```python
from build123d import *

# Parameters (mm, degrees)
FILETE1_R     = 2
CHANFRO1_SIZE = 0.5


with BuildPart() as part:
    # Esboço1 → Revolução1 (revolve)
    with BuildSketch(Plane.XY, mode=Mode.PRIVATE) as revolu_o1_sk:
        Polygon((0, 58.936157254), (12.5, 58.936157254), (12.5, 54.936157254), (6, 54.936157254), (6, 42.536157254), (4, 42.536157254), (4, 22.536157254), (1.75, 22.536157254), (1.75, 30.536157254), (0, 31.786157254), align=None)
    revolve(revolu_o1_sk.sketch.rotate(Axis((0, -51.524307863, 0), (0, 1, 0)), 90), axis=Axis((0, -51.524307863, 0), (0, 1, 0)))

    # Filete1
    filete1_edges = [part.edges().sort_by_distance(p)[0] for p in [
        (0, 54.936157254, 12.5),
        (0, 58.936157254, 12.5),
    ]]
    fillet(filete1_edges, radius=FILETE1_R - 0.0001)  # a hair under: the kernel refuses the full size

    # Chanfro1
    chanfro1_edges = [part.edges().sort_by_distance(p)[0] for p in [
        (0, 22.536157254, 4),
    ]]
    chamfer(chanfro1_edges, length=CHANFRO1_SIZE)


solid = part.part
```
Read the model definition and answer for the solid it produces. Units are mm, in the model's axes. A direction names the side the tool comes from. Give positions to 0.01 mm unless a question says otherwise; leave off trailing zeros. Write each loop counter-clockwise with the first axis right and the second up, starting at its lowest first coordinate (ties: lowest second). Pieces come first, ordered by that corner, then holes. Notation, with made-up numbers: (0.5, -24) -> (41.5, -24) arc R34 ccw to (41.5, 14) -> close; hole circle Ø7 at (-18.75, 36.5). An arc over 180 degrees is marked (long way). Answer in a Markdown table with one row per item.
1) Section A-A on y = 29.5 is taken. Give the vertices of the cut face in (x, z).
Results list:
| item | result |
|---|---|
| outline | circle Ø8 at (0, 0); hole circle Ø3.5 at (0, 0) |
2) Determine the mould class of faces 1 (the conical face through (-0.084, 31.587, -0.267)), 2 (the flat face through (5, 54.936, -5)), 3 (the cylindrical face through (3.905, 32.65, 0.867)) for opening direction Z: released by +Z, released by -Z, zero draft, split by the parting line, or undercut.
Results list:
| item | result |
|---|---|
| face 1 | undercut |
| face 2 | zero draft |
| face 3 | split by the parting line |
3) Section C-C on y = 33.5 is taken. Give the vertices of the cut face in (x, z), plus the area to 3 significant figures.
Results list:
| item | result |
|---|---|
| outline | circle Ø8 at (0, 0) |
| area | 50.3 mm^2 |
4) Each of these flat-tipped pins is pushed along its axis until it touches: pin 1 Ø6 at (x, z) = (-1, 1) entering from -Y; pin 2 Ø12 at (x, z) = (7, 7.5) entering from -Y; pin 3 Ø10 at (y, z) = (27.5, -7) entering from +X; pin 4 Ø6 at (x, y) = (-5.5, 47) entering from +Z. Where does it stop, or does it pass through?
Results list:
| item | result |
|---|---|
| pin 1 | y = 22.54 |
| pin 2 | y = 42.54 |
| pin 3 | x = 3.46 |
| pin 4 | z = 5.45 |
5) Section B-B on y = 47 is taken. Give the vertices of the cut face in (x, z), plus the area to 3 significant figures.
Results list:
| item | result |
|---|---|
| outline | circle Ø12 at (0, 0) |
| area | 113 mm^2 |
6) Straight lines are drawn through the part: line 1 (X direction, y = 25, z = 0); line 2 (Y direction, x = 5, z = -8.25); line 3 (Y direction, x = -4.75, z = -3). For each, find the intervals that lie inside material, in ascending order. Write a range as [from, to].
Results list:
| item | result |
|---|---|
| line 1 | [-4, -1.75], [1.75, 4] |
| line 2 | [54.94, 58.94] |
| line 3 | [42.54, 58.94] |
7) A tool of negligible diameter and unlimited length cuts with its end or side. For faces 4 (the cylindrical face through (1.55, 26.59, -0.81)), 5 (the flat face through (1, 22.536, 2)), from which of +Z, -Z, +X, -X, +Y, -Y can it reach the whole face along a straight path? Write none if from no direction.
Results list:
| item | result |
|---|---|
| face 4 | -Y |
| face 5 | +Z, -Z, +X, -X, -Y |
